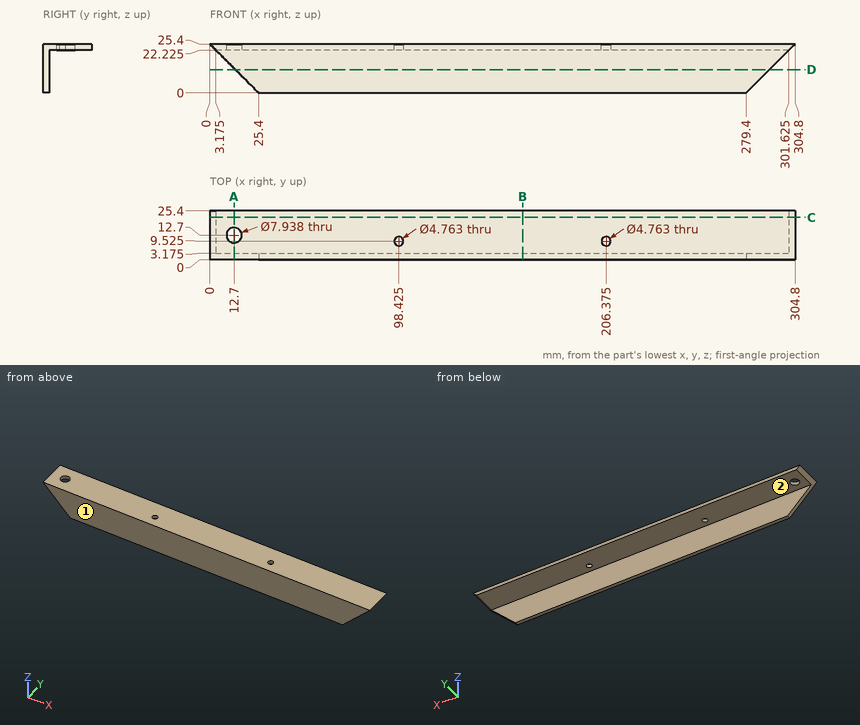
Design review of the part shown in the three views and the two pictorial views. Dimensions are in mm from the part's minimum x, y and z. A direction names the side the tool comes from. Give positions to 0.01 mm unless a question says otherwise; leave off trailing zeros. Loops run counter-clockwise (first coordinate to the right, second up) from the corner with the lowest first, then second, coordinate; pieces in that order, holes last. Notation, with made-up numbers: M 52,87 L 87,87 A37 cw 87,124 Z; hole C 13,-33.5 d8. An arc over 180 degrees is marked long. Write item = value, one per line.
Q1. We need section D-D (z = 12). Give the boundary of the cut face in (x, y) (1 decimal).
Output values:
outline = M 13.4,0 L 291.4,0 L 291.4,3.2 L 13.4,3.2 Z
Q2. We need section B-B (x = 163). Give the boundary of the cut face in (y, z) (1 decimal), plus the area to 3 significant figures.
Output values:
outline = M 0,0 L 3.2,0 L 3.2,22.2 L 25.4,22.2 L 25.4,25.4 L 0,25.4 Z
area = 151 mm^2
Q3. We need section A-A (x = 12.7). Give the boundary of the cut face in (y, z) (1 decimal).
Output values:
outline = M 0,12.7 L 3.2,12.7 L 3.2,22.2 L 8.7,22.2 L 8.7,25.4 L 0,25.4 Z; M 16.7,22.2 L 25.4,22.2 L 25.4,25.4 L 16.7,25.4 Z
Q4. Insertion check: pin 1 (12 mm diameter, centred on y = 3, z = 19, fed in from -X); pin 2 (6 mm diameter, centred on x = 69, z = 17, fed in from +Y) (1 decimal); pin 3 (7 mm diameter, centred on x = 12.7, y = 12.7, fed in from +Z); pin 4 (5 mm diameter, centred on x = 79.5, y = 11.5, fed in from -Z) (1 decimal). Each pin has a flat end and moves straight along its axis. Give the tip position at first contact, or say it passes through.
Output values:
pin_1 = 0.4
pin_2 = 3.2
pin_3 = through
pin_4 = 22.2
Q5. For the marked faces 1 and 2, list the 3-axis set-ups (+Z, -Z, +X, -X, +Y, -Y) from which the entire face can be reached by the end or side of a thin tool; tool diameter is ignored.
Output values:
face_1 = +Z, -Z, +X, -X, -Y
face_2 = -Z, +X, -X, +Y
Q6. We need section C-C (y = 22). Give the boundary of the cut face in (x, z) (1 decimal).
Output values:
outline = M 0,25.4 L 3.2,22.2 L 301.6,22.2 L 304.8,25.4 Z
Q7. To check wall thickness, follow line 1 (Y direction, x = 12.7, z = 23.7); line 2 (Z direction, x = 260.5, y = 9.75) (1 decimal); line 3 (Y direction, x = 180.5, z = 16) (1 decimal). State the ranges of each line that lie inside material, in increasing order. Write a range as [from, to].
Output values:
line_1 = [0, 8.73], [16.67, 25.4]
line_2 = [22.2, 25.4]
line_3 = [0, 3.2]
